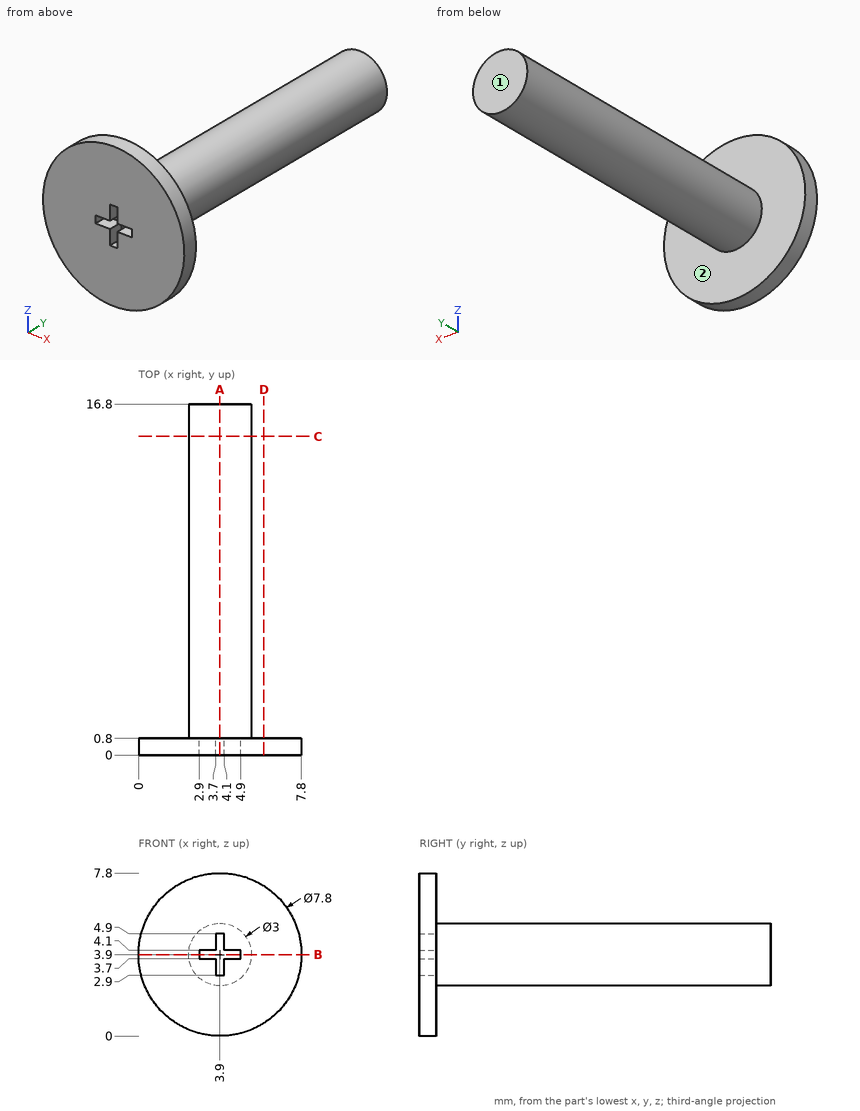
Design review of the part shown in the three views and the two pictorial views. Dimensions are in mm from the part's minimum x, y and z. A direction names the side the tool comes from. Round coordinates to 2 decimals unless told otherwise and drop trailing zeros. Loops run counter-clockwise (first coordinate to the right, second up) from the corner with the lowest first, then second, coordinate; pieces in that order, holes last.
(1) We need section B-B (z = 3.9). Give the boundary of the cut face in (x, y), plus the area to 3 significant figures.
Returned:
outline: (0, 0) - (2.9, 0) - (2.9, 0.8) - (4.9, 0.8) - (4.9, 0) - (7.8, 0) - (7.8, 0.8) - (5.4, 0.8) - (5.4, 16.8) - (2.4, 16.8) - (2.4, 0.8) - (0, 0.8) - close
area: 52.6 mm2
(2) Wall thickness on line 1 along Y through (x, z) = (3, 5.5); line 2 along Y through (x, z) = (4, 4.25); line 3 along X through (y, z) = (5.5, 2.75): over which ranges is each line inside the solid? List them lowest first.
Returned:
line 1: y = 0 to 0.8
line 2: y = 0.8 to 16.8
line 3: x = 2.94 to 4.86
(3) We need section A-A (x = 3.9). Give the boundary of the cut face in (y, z).
Returned:
outline: (0, 0) - (0.8, 0) - (0.8, 2.4) - (16.8, 2.4) - (16.8, 5.4) - (0.8, 5.4) - (0.8, 7.8) - (0, 7.8) - (0, 4.9) - (0.8, 4.9) - (0.8, 2.9) - (0, 2.9) - close
(4) Clearance check with flat-ended pins moving along their axes: P1, Ø0.9, axis at x = 3.5, y = 0, coming from the -Z side; P2, Ø0.9, axis at y = 0.5, z = 3, coming from the +X side; P3, Ø0.9, axis at x = 4.5, y = 0.5, coming from the +Z side; P4, Ø1.5, axis at y = 5, z = 5.5, coming from the -X side. State where each tip first meets the part, or that it passes through.
Returned:
P1: stops at z = 0
P2: stops at x = 7.77
P3: stops at z = 7.8
P4: stops at x = 2.66
(5) We need section C-C (y = 15.25). Give the boundary of the cut face in (x, z), plus the area to 3 significant figures.
Returned:
outline: circle Ø3 at (3.9, 3.9)
area: 7.07 mm2
(6) We need section D-D (x = 6). Give the boundary of the cut face in (y, z).
Returned:
outline: (0, 0.61) - (0.8, 0.61) - (0.8, 7.19) - (0, 7.19) - close
(7) Tool access review of the marked faces 1 and 2: name each direction out of +Z, -Z, +X, -X, +Y, -Y from which nothing blocks a thin tool from reaching the whole face with its end or side.
Returned:
face 1: +Z, -Z, +X, -X, +Y
face 2: +Y
